Check sheet for the drawn part. Datum: minimum x, y, z corner. Units: mm. A direction names the side the tool comes from. Coordinates: 2 decimals unless noted, no trailing zeros. Loops run counter-clockwise (first coordinate to the right, second up) from the corner with the lowest first, then second, coordinate; pieces in that order, holes last. Notation, with made-up numbers: (-8, -7) -> (23, -7) arc R13 cw to (23, 16) -> close; hole circle Ø11 at (11, -20). An arc over 180 degrees is marked (long way). Use CSV: the item, a comma, the result in double quotes. Start each with the question number.
1. Set-up check for the marked faces 5, 6, 7 and 8: record each of +Z, -Z, +X, -X, +Y, -Y from which the full face is reachable in a straight line by a thin tool's end or side.
2. Gauge pin test, flat ends, axial feed: pin 1 (4 mm diameter, centred on y = 6, z = 5, fed in from +X); pin 2 (1 mm diameter, centred on y = 6, z = 14, fed in from -X); pin 3 (5 mm diameter, centred on y = 6, z = 13, fed in from +X); pin 4 (2.5 mm diameter, centred on x = 9, y = 7, fed in from +Z). Record the tip position at first contact, or that the pin passes through.
3. Sectioned sample at C-C, the plane y = 2.25. Record the cut outline in (x, z), and give its area (3 significant figures).
4. Sectioned sample at D-D, the plane x = 12.5. Record the cut outline in (y, z), and give its area (3 significant figures).
5. Thickness scan on L1, parallel to Y at x = 15.2, z = 12.5; L2, parallel to X at y = 4.25, z = 10.75; L3, parallel to Y at x = 16.5, z = 22.5. Record the ranges inside material, lowest first.
6. Sectioned sample at B-B, the plane y = 7. Record the cut outline in (x, z), and give its area (3 significant figures).
7. Sectioned sample at A-A, the plane z = 12.5. Record the cut outline in (x, y).
8. Release check for a two-part mould opening along Y. For the marked faces 1, 2, 3 and 4 record: pulls with the +Y half, pulls with the -Y half, needs draft (parallel to the pull), parting line crosses it, or undercut.
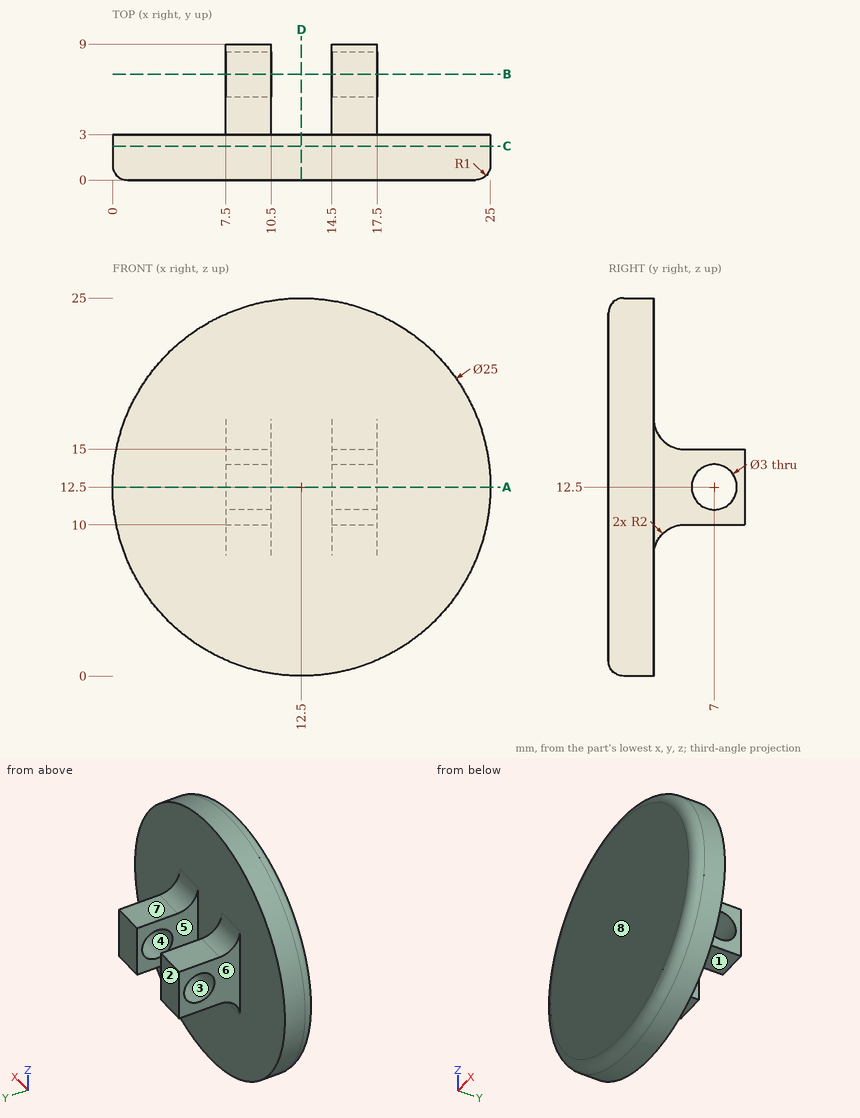
Completed:
1,face 5,"+Z, -Z, +Y"
1,face 6,"+Z, -Z, -X, +Y"
1,face 7,"+Z, +X, -X, +Y"
1,face 8,"+Z, -Z, +X, -X, -Y"
2,pin 1,"through"
2,pin 2,"x = 7.5"
2,pin 3,"x = 17.5"
2,pin 4,"z = 15"
3,outline,"circle Ø25 at (12.5, 12.5)"
3,area,"491 mm²"
4,outline,"(0, 1) arc R1 ccw to (1, 0) -> (3, 0) -> (3, 25) -> (1, 25) arc R1 ccw to (0, 24) -> close"
4,area,"74.6 mm²"
5,L1,"0 to 5.5, 8.5 to 9"
5,L2,"7.5 to 10.5, 14.5 to 17.5"
5,L3,"0 to 3"
6,outline,"(7.5, 10) -> (10.5, 10) -> (10.5, 11) -> (7.5, 11) -> close; (7.5, 14) -> (10.5, 14) -> (10.5, 15) -> (7.5, 15) -> close; (14.5, 10) -> (17.5, 10) -> (17.5, 11) -> (14.5, 11) -> close; (14.5, 14) -> (17.5, 14) -> (17.5, 15) -> (14.5, 15) -> close"
6,area,"12.0 mm²"
7,outline,"(0, 1) arc R1 ccw to (1, 0) -> (24, 0) arc R1 ccw to (25, 1) -> (25, 3) -> (17.5, 3) -> (17.5, 5.5) -> (14.5, 5.5) -> (14.5, 3) -> (10.5, 3) -> (10.5, 5.5) -> (7.5, 5.5) -> (7.5, 3) -> (0, 3) -> close; (7.5, 8.5) -> (10.5, 8.5) -> (10.5, 9) -> (7.5, 9) -> close; (14.5, 8.5) -> (17.5, 8.5) -> (17.5, 9) -> (14.5, 9) -> close"
8,face 1,"needs draft"
8,face 2,"pulls with the +Y half"
8,face 3,"undercut"
8,face 4,"undercut"
